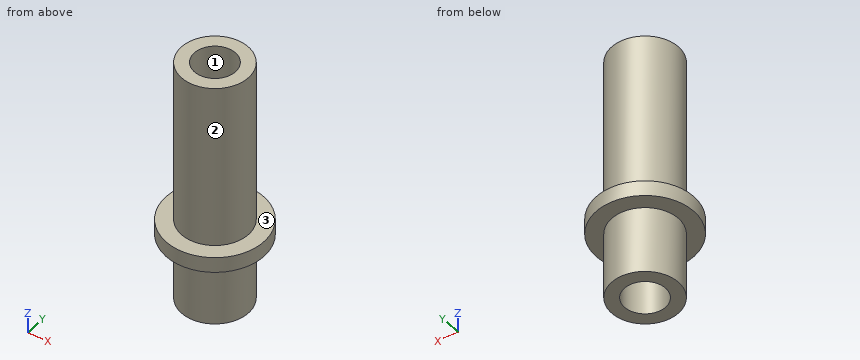
Autodesk Inventor part; units mm, degrees
ref_plane "YZ Plane" through (0, 0, 0) normal (1, 0, 0) x (0, 1, 0)
ref_plane "XZ Plane" through (0, 0, 0) normal (0, 1, 0) x (-1, 0, 0)
ref_plane "XY Plane" through (0, 0, 0) normal (0, 0, 1) x (1, 0, 0)
sketch "Skizze1" plane through (0, 0, 0) normal (0, 1, 0) x (-1, 0, 0)
  line L0 (0, 0) -> (3.25, 0)
  line L1 (3.25, 0) -> (3.25, -16)
  line L2 (3.25, -16) -> (4.75, -16)
  line L3 (4.75, -16) -> (4.75, -17.5)
  line L4 (4.75, -17.5) -> (3.25, -17.5)
  line L5 (3.25, -17.5) -> (3.25, -24)
  line L6 (3.25, -24) -> (0, -24)
  line L7 (0, -24) -> (0, 0)
  point P0 (4.75, -16.75)
  dimension "d0" = 6.5
  dimension "d1" = 9.5
  dimension "d2" = 16
  dimension "d3" = 1.5
  dimension "d4" = 6.5
revolve "Umdrehung1" add sketch "Skizze1" angle 360 about axis through (0, 0, -24) along (0, 0, 1)
sketch "Skizze2" plane through (0, 0, -24) normal (0, 0, -1) x (-1, 0, 0)
  circle A0 centre (0, 0) radius 3.25
hole "Bohrung1" at (0, 0, -24) direction (0, 0, 1) diameter 4 depth 24
properties part number "07" material "Nylon 6/6"
Build history of the part. All positions in model axes, mm. Face numbers are marked on the shaded views. Give positions to 0.01 mm unless a question says otherwise; leave off trailing zeros. Loops run counter-clockwise (first coordinate to the right, second up) from the corner with the lowest first, then second, coordinate; pieces in that order, holes last. Notation, with made-up numbers: (-13, 47) - (10, 47) arc R15 cw to (10, 56) - close; hole circle Ø8 at (15, 78). An arc over 180 degrees is marked (long way). Use a Markdown table: item, result.
(1) Band-saw the part on C-C (z = -11.75). Give the cut face in (x, y).
Taken from the geometry:
| item | result |
|---|---|
| outline | circle Ø6.5 at (0, 0); hole circle Ø4 at (0, 0) |
(2) Band-saw the part on D-D (x = -2.5). Give the cut face in (y, z).
Taken from the geometry:
| item | result |
|---|---|
| outline | (-4.04, -17.5) - (-2.08, -17.5) - (-2.08, -24) - (2.08, -24) - (2.08, -17.5) - (4.04, -17.5) - (4.04, -16) - (2.08, -16) - (2.08, 0) - (-2.08, 0) - (-2.08, -16) - (-4.04, -16) - close |
(3) Wall check: line 1 along Y through (x, z) = (0, -16.75); line 2 along Y through (x, z) = (0, -19). Give the ranges that are in metal, low to high.
Taken from the geometry:
| item | result |
|---|---|
| line 1 | -4.75 to -2, 2 to 4.75 |
| line 2 | -3.25 to -2, 2 to 3.25 |
(4) Pull direction X, two halves, no side cores. Call the marked faces 1, 2 and 3: +X half, -X half, draft (parallel to the pull), parting line (faces both ways), or undercut.
Taken from the geometry:
| item | result |
|---|---|
| face 1 | undercut |
| face 2 | parting line |
| face 3 | draft |
(5) Band-saw the part on A-A (x = 0). Give the cut face in (y, z).
Taken from the geometry:
| item | result |
|---|---|
| outline | (-4.75, -17.5) - (-3.25, -17.5) - (-3.25, -24) - (-2, -24) - (-2, 0) - (-3.25, 0) - (-3.25, -16) - (-4.75, -16) - close; (2, -24) - (3.25, -24) - (3.25, -17.5) - (4.75, -17.5) - (4.75, -16) - (3.25, -16) - (3.25, 0) - (2, 0) - close |
